Verification items for the finished model (mm, model axes). Face numbers are marked on the shaded views. A direction names the side the tool comes from. Give positions to 0.01 mm unless a question says otherwise; leave off trailing zeros. Loops run counter-clockwise (first coordinate to the right, second up) from the corner with the lowest first, then second, coordinate; pieces in that order, holes last. Notation, with made-up numbers: (-33, 76.5) -> (-17, 76.5) arc R28 ccw to (-17, 105.5) -> close; hole circle Ø11 at (72, 58). An arc over 180 degrees is marked (long way). Answer in a Markdown table with one row per item. Add a question column.
Q1. Section check C-C on y = 0.35. Enter the section's corners in (x, z).
Q2. Set-up check for the marked faces 1 and 2: record each of +Z, -Z, +X, -X, +Y, -Y from which the full face is reachable in a straight line by a thin tool's end or side.
Q3. Gauge pin test, flat ends, axial feed: P1, Ø3, axis at x = -2, z = 8, coming from the +Y side; P2, Ø1, axis at x = 2, z = 25.5, coming from the +Y side; P3, Ø1.5, axis at x = 0, y = 0, coming from the +Z side; P4, Ø1.5, axis at y = -0.5, z = 26, coming from the +X side. Record the tip position at first contact, or that the pin passes through.
Q4. Section check B-B on z = 9.5. Enter the section's corners in (x, y).
Q5. Material ranges on probe 1 along Y at (x, z) = (0, 30.3); probe 2 along Z at (x, y) = (-1.2, -1.3); probe 3 along X at (y, z) = (1.05, 29), recorded low to high.
Q6. Section check A-A on x = 0. Enter the section's corners in (y, z), and give its area (3 significant figures).
Q7. Section check D-D on x = -2.05. Enter the section's corners in (y, z).
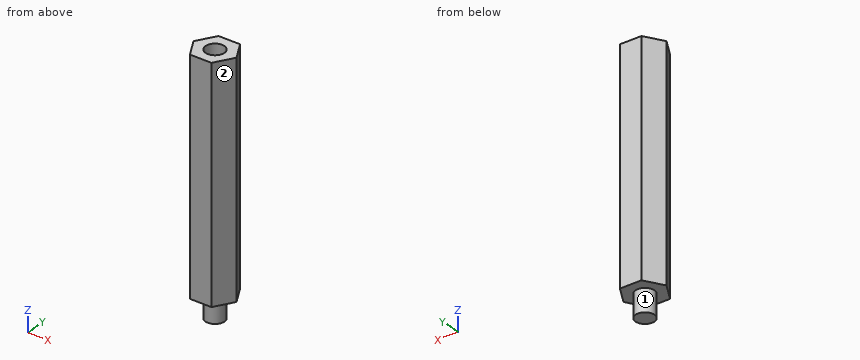
```python
from build123d import *

# Parameters (mm, degrees)
F0_R     = 1.25
F1_DEPTH = 1.5
F2_R     = 1.25
F3_DEPTH = 30
F4_R     = 1.25
F5_DEPTH = 3


with BuildPart() as f1:
    # F0 (on Top) → F1 (new body, symmetric)
    with BuildSketch(Plane.XY):
        Circle(F0_R)
    extrude(amount=F1_DEPTH, both=True)

    # F2 (on face) → F3 (join)
    with BuildSketch(Plane.XY.offset(1.5)):
        Polygon((-1.443375673, -2.5), (1.443375673, -2.5), (2.8867513459, 0), (1.443375673, 2.5), (-1.443375673, 2.5), (-2.8867513459, 0), align=None)
        Circle(F2_R, mode=Mode.SUBTRACT)
        Circle(F2_R)
    extrude(amount=F3_DEPTH)

    # F4 (on face) → F5 (cut)
    with BuildSketch(Plane.XY.offset(31.5)):
        Circle(F4_R)
    extrude(amount=-F5_DEPTH, mode=Mode.SUBTRACT)


solid = f1.part
```
Taken from the geometry:
| question | item | result |
|---|---|---|
| 1 | outline | (-2.68, 1.5) -> (-1.2, 1.5) -> (-1.2, -1.5) -> (1.2, -1.5) -> (1.2, 1.5) -> (2.68, 1.5) -> (2.68, 31.5) -> (1.2, 31.5) -> (1.2, 28.5) -> (-1.2, 28.5) -> (-1.2, 31.5) -> (-2.68, 31.5) -> close |
| 2 | face 1 | -Z |
| 2 | face 2 | +Z, -Z, +X, -Y |
| 3 | P1 | stops at y = 2.5 |
| 3 | P2 | stops at y = 2.4 |
| 3 | P3 | stops at z = 28.5 |
| 3 | P4 | stops at x = 2.89 |
| 4 | outline | (-2.89, 0) -> (-1.44, -2.5) -> (1.44, -2.5) -> (2.89, 0) -> (1.44, 2.5) -> (-1.44, 2.5) -> close |
| 5 | probe 1 | y = -2.5 to -1.25, 1.25 to 2.5 |
| 5 | probe 2 | z = 1.5 to 31.5 |
| 5 | probe 3 | x = -2.28 to -0.68, 0.68 to 2.28 |
| 6 | outline | (-2.5, 1.5) -> (-1.25, 1.5) -> (-1.25, -1.5) -> (1.25, -1.5) -> (1.25, 1.5) -> (2.5, 1.5) -> (2.5, 31.5) -> (1.25, 31.5) -> (1.25, 28.5) -> (-1.25, 28.5) -> (-1.25, 31.5) -> (-2.5, 31.5) -> close |
| 6 | area | 150 mm² |
| 7 | outline | (-1.45, 1.5) -> (1.45, 1.5) -> (1.45, 31.5) -> (-1.45, 31.5) -> close |
